The listing builds one solid part. Answer for the finished solid, in the listing's coordinates (mm). A direction names the side the tool comes from. Coordinates: 2 decimals unless noted, no trailing zeros. Write each loop counter-clockwise with the first axis right and the second up, starting at its lowest first coordinate (ties: lowest second). Pieces come first, ordered by that corner, then holes. Notation, with made-up numbers: M 86,-14.75 L 101,-14.75 A14 ccw 101,7.25 Z; hole C -17,47 d11. An arc over 180 degrees is marked long. Write item = value, one per line. Start each with the question number.
```python
from build123d import *

# Parameters (mm, degrees)
SKETCH1_W           = 762
SKETCH1_H           = 234.95
BOSS_EXTRUDE1_DEPTH = 12.7
SKETCH2_W           = 38.1
SKETCH2_H           = 38.1
BOSS_EXTRUDE2_DEPTH = 70
SKETCH3_W           = 165.1
SKETCH3_H           = 234.95
BOSS_EXTRUDE3_DEPTH = 6.35
SKETCH4_W           = 100
SKETCH4_H           = 50
SKETCH4_W_2         = 112.7
BOSS_EXTRUDE4_DEPTH = 5


with BuildPart() as part:
    # Sketch1 → Boss-Extrude1 (new body, symmetric)
    with BuildSketch(Plane(origin=(0, 0, 0), x_dir=(1, 0, 0), z_dir=(0, 1, 0))):
        with Locations((192.9, 0)):
            Rectangle(SKETCH1_W, SKETCH1_H)
    extrude(amount=BOSS_EXTRUDE1_DEPTH, both=True)

    # Sketch2 → Boss-Extrude2 (add)
    with BuildSketch(Plane(origin=(0, 12.7, 0), x_dir=(1, 0, 0), z_dir=(0, 1, 0))):
        with Locations((554.85, 98.425)):
            Rectangle(SKETCH2_W, SKETCH2_H)
        with Locations((554.85, -98.425)):
            Rectangle(SKETCH2_W, SKETCH2_H)
        with Locations((440.55, -98.425)):
            Rectangle(SKETCH2_W, SKETCH2_H)
        with Locations((440.55, 98.425)):
            Rectangle(SKETCH2_W, SKETCH2_H)
    extrude(amount=BOSS_EXTRUDE2_DEPTH)

    # Sketch3 → Boss-Extrude3 (add)
    with BuildSketch(Plane(origin=(0, 82.7, 0), x_dir=(1, 0, 0), z_dir=(0, 1, 0))):
        with Locations((491.35, 0)):
            Rectangle(SKETCH3_W, SKETCH3_H)
    extrude(amount=BOSS_EXTRUDE3_DEPTH)

    # Sketch4 → Boss-Extrude4 (add)
    with BuildSketch(Plane(origin=(0, 12.7, 0), x_dir=(1, 0, 0), z_dir=(0, 1, 0))):
        with Locations((-138.1, 67.75)):
            Rectangle(SKETCH4_W, SKETCH4_H)
        with Locations((-131.75, -67.75)):
            Rectangle(SKETCH4_W_2, SKETCH4_H)
    extrude(amount=BOSS_EXTRUDE4_DEPTH)


solid = part.part
```
1. For faces 1 (the face through (188, 12.7, -2)), 2 (the face through (-133, 17.7, 67)), 3 (the face through (459.6, 47, 99)), determine the directions among +Z, -Z, +X, -X, +Y, -Y from which every point of the face is accessible in a straight line to the end or side of a thin tool.
2. Each of these flat-tipped pins is pushed along its axis until it touches: pin 1 (2.5 mm diameter, centred on x = -145, y = 15, fed in from -Z); pin 2 (10 mm diameter, centred on x = -47.5, z = -6.5, fed in from +Y); pin 3 (25 mm diameter, centred on x = -148, z = 79.5, fed in from +Y). Where does it stop, or does it pass through?
3. The part is cut by section D-D, the plane z = 10.5. Write down the section's boundary in (x, y), and give its area (3 significant figures).
4. The part is cut by section A-A, the plane x = 503. Write down the section's boundary in (y, z) (3 decimals).
5. For a pull along X with two mould halves and no side action, classify faces 4 (the face through (573.9, 4, 28)), 5 (the face through (-139, 17.7, -68)), 6 (the face through (490, 82.7, -2)) as pulls with the +X half, pulls with the -X half, needs draft (parallel to the pull), parting line crosses it, or undercut.
6. The part is cut by section B-B, the plane z = 67. Write down the section's boundary in (x, y), and give its area (3 significant figures).
7. Straight lines are drawn through the part: L1, parallel to Y at x = 410.5, z = 84.5; L2, parallel to X at y = 66, z = 80.5; L3, parallel to Y at x = 398, z = 99. For each, find the intervals that lie inside material, in ascending order. Write a range as [from, to].
8. The part is cut by section C-C, the plane y = 55.5. Write down the section's boundary in (x, z) (3 decimals).
Solution:
q1.face_1 = none
q1.face_2 = +Z, -Z, -X, +Y
q1.face_3 = +Z, -Z
q2.pin_1 = -92.75
q2.pin_2 = 12.7
q2.pin_3 = 17.7
q3.outline = M -188.1,-12.7 L 573.9,-12.7 L 573.9,12.7 L -188.1,12.7 Z; M 408.8,82.7 L 573.9,82.7 L 573.9,89.05 L 408.8,89.05 Z
q3.area = 20,400 mm^2
q4.outline = M -12.7,-117.475 L 12.7,-117.475 L 12.7,117.475 L -12.7,117.475 Z; M 82.7,-117.475 L 89.05,-117.475 L 89.05,117.475 L 82.7,117.475 Z
q5.face_4 = pulls with the +X half
q5.face_5 = needs draft
q5.face_6 = undercut
q6.outline = M -188.1,-12.7 L 573.9,-12.7 L 573.9,12.7 L -75.4,12.7 L -75.4,17.7 L -188.1,17.7 Z; M 408.8,82.7 L 573.9,82.7 L 573.9,89.05 L 408.8,89.05 Z
q6.area = 21,000 mm^2
q7.L1 = [-12.7, 12.7], [82.7, 89.05]
q7.L2 = [421.5, 459.6], [535.8, 573.9]
q7.L3 = [-12.7, 12.7]
q8.outline = M 421.5,-117.475 L 459.6,-117.475 L 459.6,-79.375 L 421.5,-79.375 Z; M 421.5,79.375 L 459.6,79.375 L 459.6,117.475 L 421.5,117.475 Z; M 535.8,-117.475 L 573.9,-117.475 L 573.9,-79.375 L 535.8,-79.375 Z; M 535.8,79.375 L 573.9,79.375 L 573.9,117.475 L 535.8,117.475 Z
